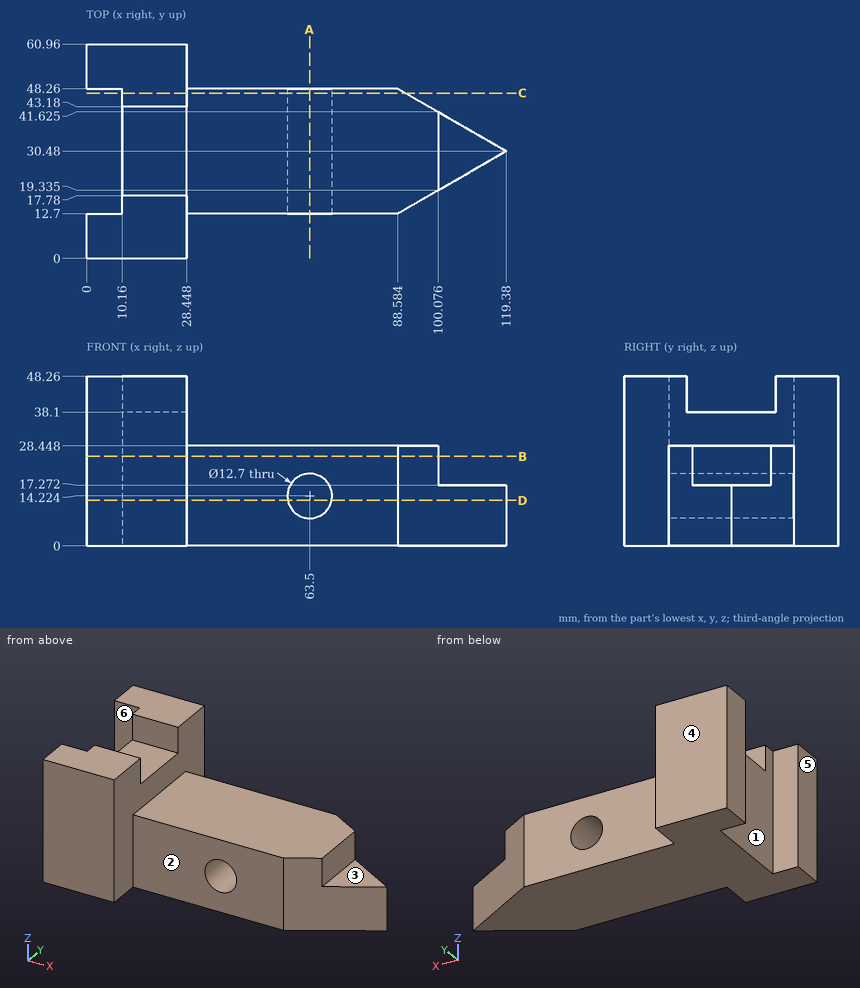
Check sheet for the drawn part. Datum: minimum x, y, z corner. Units: mm. A direction names the side the tool comes from. Round coordinates to 2 decimals unless told otherwise and drop trailing zeros. Write each loop counter-clockwise with the first axis right and the second up, starting at its lowest first coordinate (ties: lowest second). Pieces come first, ordered by that corner, then holes. Notation, with made-up numbers: (-26, -14.75) -> (7, -14.75) arc R24 cw to (7, 6.25) -> close; hole circle Ø4 at (81, -28). An arc over 180 degrees is marked (long way). Put each result on its own line as item: value.
(1) Mould release check, pull along Y, two halves, no side actions. Record for the marked faces 4, 5 and 6: released by +Y, released by -Y, zero draft, split by the parting line, or undercut.
Values found:
face 4: released by +Y
face 5: zero draft
face 6: undercut
(2) Tool access check on the marked faces 1, 2 and 3. Record the directions out of +Z, -Z, +X, -X, +Y, -Y that give a thin tool (end or side, any length) a straight path to the whole face; none if there is none.
Values found:
face 1: +Z, -Z, -X
face 2: +Z, -Z, +X, -Y
face 3: +Z, +X, +Y, -Y
(3) Go/stop test with flat-tipped pins: pin 1 Ø14.5 at (y, z) = (38, 31) entering from +X; pin 2 Ø14.5 at (x, y) = (18, 35) entering from +Z; pin 3 Ø1 at (x, y) = (35.5, 46) entering from +Z. Record where each tip stops, or that it passes through.
Values found:
pin 1: stops at x = 100.08
pin 2: stops at z = 38.1
pin 3: stops at z = 28.45
(4) Sectioned sample at D-D (z = 13). Enter the section's corners in (x, y), plus the area to 3 significant figures.
Values found:
outline: (0, 0) -> (28.45, 0) -> (28.45, 12.7) -> (57.27, 12.7) -> (57.27, 48.26) -> (28.45, 48.26) -> (28.45, 60.96) -> (0, 60.96) -> (0, 48.26) -> (10.16, 48.26) -> (10.16, 12.7) -> (0, 12.7) -> close; (69.73, 12.7) -> (88.58, 12.7) -> (119.38, 30.48) -> (88.58, 48.26) -> (69.73, 48.26) -> close
area: 3,620 mm^2
(5) Sectioned sample at A-A (x = 63.5). Enter the section's corners in (y, z), plus the area to 3 significant figures.
Values found:
outline: (12.7, 0) -> (48.26, 0) -> (48.26, 7.87) -> (12.7, 7.87) -> close; (12.7, 20.57) -> (48.26, 20.57) -> (48.26, 28.45) -> (12.7, 28.45) -> close
area: 560 mm^2
(6) Material ranges on line 1 (Y direction, x = 27, z = 42); line 2 (Z direction, x = 63, y = 36); line 3 (Y direction, x = 10, z = 35.5), recorded low to high.
Values found:
line 1: y = 0 to 17.78, 43.18 to 60.96
line 2: z = 0 to 7.89, 20.55 to 28.45
line 3: y = 0 to 12.7, 48.26 to 60.96
(7) Sectioned sample at C-C (y = 47). Enter the section's corners in (x, z).
Values found:
outline: (10.16, 0) -> (90.77, 0) -> (90.77, 28.45) -> (28.45, 28.45) -> (28.45, 48.26) -> (10.16, 48.26) -> close; hole circle Ø12.7 at (63.5, 14.22)
(8) Sectioned sample at B-B (z = 25.5). Enter the section's corners in (x, y) (1 decimal).
Values found:
outline: (0, 0) -> (28.4, 0) -> (28.4, 12.7) -> (88.6, 12.7) -> (100.1, 19.3) -> (100.1, 41.6) -> (88.6, 48.3) -> (28.4, 48.3) -> (28.4, 61) -> (0, 61) -> (0, 48.3) -> (10.2, 48.3) -> (10.2, 12.7) -> (0, 12.7) -> close
